Input: part model. Units: mm. Frame: model coordinates. Give positions to 0.01 mm unless a question says otherwise; leave off trailing zeros. Loops run counter-clockwise (first coordinate to the right, second up) from the corner with the lowest first, then second, coordinate; pieces in that order, holes last. Notation, with made-up numbers: (31.5, -0.5) -> (64.5, -0.5) arc R23 ccw to (64.5, 13.5) -> close; hole circle Ø1 at (16, 43.25). An arc over 180 degrees is marked (long way). Answer as a JSON object with one key per item and string values.
```python
from build123d import *

# Parameters (mm, degrees)
SKETCH1_W           = 43.2
SKETCH1_H           = 18
BOSS_EXTRUDE2_DEPTH = 1.6
SKETCH2_R           = 0.45
CUT_EXTRUDE2_DEPTH  = 1.6
LPATTERN1_COUNT     = 15
LPATTERN1_PITCH     = 2.54
SKETCH3_R           = 0.5
CUT_EXTRUDE4_DEPTH  = 1.6
SKETCH4_R           = 0.9
CUT_EXTRUDE5_DEPTH  = 1.6
SKETCH9_R           = 0.4
CUT_EXTRUDE6_DEPTH  = 10


with BuildPart() as part:
    # Sketch1 → Boss-Extrude2 (new body)
    with BuildSketch(Plane(origin=(0, 0, 0), x_dir=(1, 0, 0), z_dir=(0, 1, 0))):
        with Locations((17.78, 7.62)):
            Rectangle(SKETCH1_W, SKETCH1_H)
    extrude(amount=BOSS_EXTRUDE2_DEPTH)

    # Sketch2 → Cut-Extrude2 (cut)
    with BuildSketch(Plane(origin=(0, 0, 0), x_dir=(1, 0, 0), z_dir=(0, 1, 0))):
        Circle(SKETCH2_R)
        with Locations((0, 15.24)):
            Circle(SKETCH2_R)
    cut_extrude2 = extrude(amount=CUT_EXTRUDE2_DEPTH, mode=Mode.SUBTRACT)

    # LPattern1: Cut-Extrude2 ×15
    with Locations(*[(i * LPATTERN1_PITCH, 0, 0) for i in range(1, LPATTERN1_COUNT)]):
        add(cut_extrude2, mode=Mode.SUBTRACT)

    # Sketch3 → Cut-Extrude4 (cut)
    with BuildSketch(Plane(origin=(0, 0, 0), x_dir=(1, 0, 0), z_dir=(0, 1, 0))):
        with Locations((0.127, 10.16)):
            Circle(SKETCH3_R)
        with Locations((-2.413, 10.16)):
            Circle(SKETCH3_R)
        with Locations((-2.413, 7.62)):
            Circle(SKETCH3_R)
        with Locations((-2.413, 5.08)):
            Circle(SKETCH3_R)
        with Locations((0.127, 5.08)):
            Circle(SKETCH3_R)
        with Locations((0.127, 7.62)):
            Circle(SKETCH3_R)
    extrude(amount=CUT_EXTRUDE4_DEPTH, mode=Mode.SUBTRACT)

    # Sketch4 → Cut-Extrude5 (cut)
    with BuildSketch(Plane(origin=(0, 0, 0), x_dir=(1, 0, 0), z_dir=(0, 1, 0))):
        with Locations((38.1, 15.24)):
            Circle(SKETCH4_R)
        with Locations((38.1, 0)):
            Circle(SKETCH4_R)
        with Locations((-2.54, 0)):
            Circle(SKETCH4_R)
        with Locations((-2.54, 15.24)):
            Circle(SKETCH4_R)
    extrude(amount=CUT_EXTRUDE5_DEPTH, mode=Mode.SUBTRACT)

    # Sketch9 → Cut-Extrude6 (cut)
    with BuildSketch(Plane(origin=(0, 0, 0), x_dir=(1, 0, 0), z_dir=(0, 1, 0))):
        with Locations((35.33, 5.42)):
            Circle(SKETCH9_R)
        with Locations((35.33, 9.82)):
            Circle(SKETCH9_R)
    extrude(amount=CUT_EXTRUDE6_DEPTH, mode=Mode.SUBTRACT)


solid = part.part
```
Q1. Draft query along X for faces 1 (the flat face through (17, 1, -16.62)), 2 (the cylindrical face through (19.87, 0.79, -15.26)), 3 (the cylindrical face through (35.7, 0.79, -9.67)), 4 (the flat face through (39.38, 1, -7)). Return one class per face: +X half, -X half, draft (parallel to the pull), parting line (faces both ways), or undercut.
Evaluation:
{"face 1": "draft", "face 2": "undercut", "face 3": "undercut", "face 4": "+X half"}
Q2. Section C-C, the plane x = 7.62. Return the cut outline in (y, z), then the cut area to 3 significant figures.
Evaluation:
{"outline": "(0, -16.62) -> (1.6, -16.62) -> (1.6, -15.69) -> (0, -15.69) -> close; (0, -14.79) -> (1.6, -14.79) -> (1.6, -0.45) -> (0, -0.45) -> close; (0, 0.45) -> (1.6, 0.45) -> (1.6, 1.38) -> (0, 1.38) -> close", "area": "25.9 mm2"}
Q3. Section A-A, the plane x = 38.1. Return the cut outline in (y, z), then the cut area to 3 significant figures.
Evaluation:
{"outline": "(0, -16.62) -> (1.6, -16.62) -> (1.6, -16.14) -> (0, -16.14) -> close; (0, -14.34) -> (1.6, -14.34) -> (1.6, -0.9) -> (0, -0.9) -> close; (0, 0.9) -> (1.6, 0.9) -> (1.6, 1.38) -> (0, 1.38) -> close", "area": "23.0 mm2"}
Q4. Ray query, line 1 along Z through (x, y) = (15.24, 1); line 2 along X through (y, z) = (0.8, -8); line 3 along X through (y, z) = (0.95, -0.75). Return the intervals inside material, ascending.
Evaluation:
{"line 1": "z = -16.62 to -15.69, -14.79 to -0.45, 0.45 to 1.38", "line 2": "x = -3.82 to -2.74, -2.09 to -0.2, 0.45 to 39.38", "line 3": "x = -3.82 to -3.04, -2.04 to 37.6, 38.6 to 39.38"}
Q5. Section B-B, the plane z = 0. Give the number of separate pieces and of enclosed holes in the cut face, then the cut area to 3 significant figures.
Evaluation:
{"separate pieces": "18", "enclosed holes": "0", "area": "41.8 mm2"}
Q6. Pin query (flat end, axial travel): pin 1 (1.4 mm diameter, centred on x = 38.1, z = 0, fed in from -Y). Return the tip coordinate at first contact, or that it passes through.
Evaluation:
{"pin 1": "passes through"}
